from build123d import *

# Parameters (mm, degrees)
BOSS_EXTRUDE1_DEPTH = 5


with BuildPart() as part:
    # Sketch3 → Boss-Extrude1 (new body)
    with BuildSketch(Plane.XY.offset(4.376601216)):
        Polygon((-41.095887165, 37.669622361), (-13.754633765, -1.155465661), (24.040364141, 2.253439084), (21.87007244, 26.315763035), (-3.700822745, 24.009406354), (-22.528508458, 50.745070018), (-26.12981396, 48.208972579), (-23.826719635, 44.93853583), (-22.641186314, 45.773407523), (-20.91386557, 43.320579961), (-22.099398891, 42.485708268), (-18.644757404, 37.580053144), (-21.833433235, 35.334536178), (-25.288074722, 40.240191301), (-26.473608044, 39.405319609), (-28.200928787, 41.85814717), (-27.015395466, 42.693018863), (-29.318489791, 45.963455612), (-34.305905833, 42.451236767), (-32.002811508, 39.180800018), (-30.817278187, 40.015671711), (-29.089957443, 37.562844149), (-30.275490764, 36.727972456), (-26.820849277, 31.822317332), (-30.009525108, 29.576800365), (-33.464166595, 34.482455489), (-34.649699917, 33.647583796), (-36.37702066, 36.100411358), (-35.191487339, 36.935283051), (-37.494581664, 40.2057198), align=None)
        Polygon((3.674129189, 16.601950475), (4.399955221, 8.554616968), (11.732063487, 5.159533997), (18.338345721, 9.811784534), (17.612519688, 17.859118041), (10.280411422, 21.254201011), align=None, mode=Mode.SUBTRACT)
    extrude(amount=-BOSS_EXTRUDE1_DEPTH)


solid = part.part
For this review, take the finished solid that the model builds, in its own axes (mm). A direction names the side the tool comes from. Round coordinates to 2 decimals unless told otherwise and drop trailing zeros. Order: outer loops, then holes, each group sorted by start corner. A loop starts at its lowest first (then second) coordinate and runs counter-clockwise, first axis right, second up. Notation, with made-up numbers: M 48.25,84.25 L 92.25,84.25 A26 ccw 92.25,108.25 Z; hole C 11.25,62.25 d2. An arc over 180 degrees is marked long. Use a Markdown table: item, result. Add a question column.
Item 1: To check wall thickness, follow line 1 along X through (y, z) = (36.5, 0.8); line 2 along Y through (x, z) = (-22, 1.2); line 3 along X through (y, z) = (5.5, 1.15). State the ranges of each line that lie inside material, in increasing order.
Item 2: Add section D-D, the plane x = -8. Give the boundary of the cut face in (y, z).
Item 3: Tool access review of faces 1 (the flat face through (-9, 19, 4.377)), 2 (the flat face through (-28.151, 44.305, 1.912)), 3 (the flat face through (17.98, 13.78, 1.91)): name each direction out of +Z, -Z, +X, -X, +Y, -Y from which nothing blocks a thin tool from reaching the whole face with its end or side.
Item 4: Add section C-C, the plane y = 38.5. Give the boundary of the cut face in (x, z), then the cut area to 3 significant figures.
Item 5: Insertion check: pin 1 (3 mm diameter, centred on y = 30.5, z = 0.5, fed in from -X); pin 2 (2 mm diameter, centred on y = 11.5, z = 1.5, fed in from -X); pin 3 (1 mm diameter, centred on x = -33.5, z = 1, fed in from +Y). Each pin has a flat end and moves straight along its axis. Give the tip position at first contact, or say it passes through.
Item 6: Mouldability with a two-part tool opening along X and no side actions: class faces 4 (the flat face through (-39.27, 38.955, 1.912)), 5 (the flat face through (22.97, 14.12, 1.91)), 6 (the flat face through (-20.4, 40.07, 1.91)), 7 (the flat face through (-23.537, 37.753, 1.912)) as released by +X, released by -X, zero draft, split by the parting line, or undercut.
Item 7: Add section A-A, the plane y = 15.5. Give the boundary of the cut face in (x, z).
Item 8: Add section B-B, the plane x = 9. Give the boundary of the cut face in (y, z).
Geometry results:
| question | item | result |
|---|---|---|
| 1 | line 1 | x = -40.27 to -35.81, -30.11 to -22.65, -20.18 to -12.5 |
| 1 | line 2 | y = 10.55 to 35.57, 42.34 to 42.56, 44.86 to 49.99 |
| 1 | line 3 | x = -18.44 to 11, 12.22 to 23.75 |
| 2 | outline | M -0.64,-0.62 L 30.11,-0.62 L 30.11,4.38 L -0.64,4.38 Z |
| 3 | face 1 | +Z, +X, -X, +Y, -Y |
| 3 | face 2 | +Z, -Z, +Y |
| 3 | face 3 | +Z, -Z |
| 4 | outline | M -39.92,-0.62 L -36.29,-0.62 L -36.29,4.38 L -39.92,4.38 Z; M -29.75,-0.62 L -24.06,-0.62 L -24.06,4.38 L -29.75,4.38 Z; M -19.29,-0.62 L -13.91,-0.62 L -13.91,4.38 L -19.29,4.38 Z |
| 4 | area | 73.5 mm² |
| 5 | pin 1 | stops at x = -37.1 |
| 5 | pin 2 | stops at x = -23.37 |
| 5 | pin 3 | stops at y = 43.37 |
| 6 | face 4 | released by -X |
| 6 | face 5 | released by +X |
| 6 | face 6 | undercut |
| 6 | face 7 | undercut |
| 7 | outline | M -25.48,-0.62 L 3.77,-0.62 L 3.77,4.38 L -25.48,4.38 Z; M 17.83,-0.62 L 22.85,-0.62 L 22.85,4.38 L 17.83,4.38 Z |
| 8 | outline | M 0.9,-0.62 L 6.42,-0.62 L 6.42,4.38 L 0.9,4.38 Z; M 20.35,-0.62 L 25.15,-0.62 L 25.15,4.38 L 20.35,4.38 Z |
